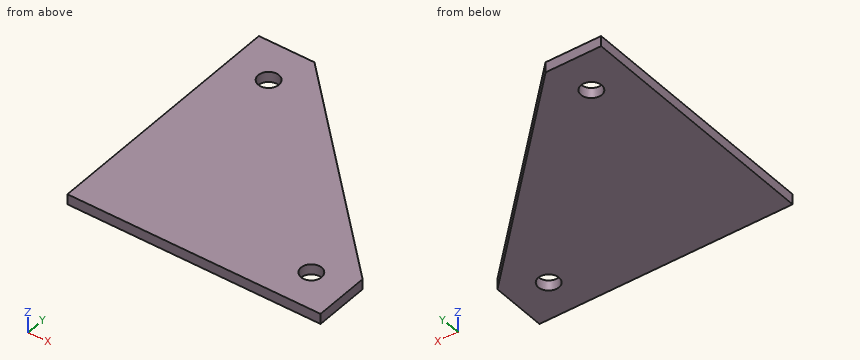
```python
from build123d import *

# Parameters (mm, degrees)
F0_R     = 1.5875
F1_DEPTH = 0.79375


with BuildPart() as f1:
    # F0 (on Top) → F1 (new body, symmetric)
    with BuildSketch(Plane.XY):
        Polygon((-33.090407, 33.090407), (-33.090407, -5.813425), (5.813425, -5.813425), (5.813425, 2.72617), (-24.550812, 33.090407), align=None)
        Circle(F0_R, mode=Mode.SUBTRACT)
        with Locations((-26.940768, 26.940768)):
            Circle(F0_R, mode=Mode.SUBTRACT)
    extrude(amount=F1_DEPTH, both=True)


solid = f1.part
```
Verification items for the finished model (mm, model axes). Round coordinates to 2 decimals unless told otherwise and drop trailing zeros. Loops run counter-clockwise (first coordinate to the right, second up) from the corner with the lowest first, then second, coordinate; pieces in that order, holes last. Notation, with made-up numbers: (29, -18) -> (44, -18) arc R9 cw to (44, -2) -> close; hole circle Ø8 at (41, -36). An arc over 180 degrees is marked (long way). Answer as a JSON object with one key per item and string values.
Q1. Scan lines: line 1 (Y direction, x = -1, z = -0.55); line 2 (Y direction, x = 0, z = 0.35); line 3 (Y direction, x = -20, z = 0.1). Record each from-to range of solid material in increasing order. Write a range as from..to.
Data:
{"line 1": "y = -5.81..-1.23, 1.23..9.54", "line 2": "y = -5.81..-1.59, 1.59..8.54", "line 3": "y = -5.81..28.54"}
Q2. Section check A-A (y = 0). Record the boundary of the cut face in (x, z), then the cut area to 3 significant figures.
Data:
{"outline": "(-33.09, -0.79) -> (-1.59, -0.79) -> (-1.59, 0.79) -> (-33.09, 0.79) -> close; (1.59, -0.79) -> (5.81, -0.79) -> (5.81, 0.79) -> (1.59, 0.79) -> close", "area": "56.7 mm2"}
Q3. Section check B-B (z = 0.05). Record the boundary of the cut face in (x, y) (1 decimal).
Data:
{"outline": "(-33.1, -5.8) -> (5.8, -5.8) -> (5.8, 2.7) -> (-24.6, 33.1) -> (-33.1, 33.1) -> close; hole circle Ø3.2 at (-26.9, 26.9); hole circle Ø3.2 at (0, 0)"}
Q4. Go/stop test with a flat-tipped pin: P1, Ø3, axis at x = -26.94, y = 26.94, coming from the +Z side. Record where the tip stops, or that it passes through.
Data:
{"P1": "passes through"}
Q5. Section check C-C (x = -26). Record the boundary of the cut face in (y, z).
Data:
{"outline": "(-5.81, -0.79) -> (25.66, -0.79) -> (25.66, 0.79) -> (-5.81, 0.79) -> close; (28.22, -0.79) -> (33.09, -0.79) -> (33.09, 0.79) -> (28.22, 0.79) -> close"}
Q6. Section check D-D (y = 8). Record the boundary of the cut face in (x, z).
Data:
{"outline": "(-33.09, -0.79) -> (0.54, -0.79) -> (0.54, 0.79) -> (-33.09, 0.79) -> close"}
